from build123d import *

# Parameters (mm, degrees)
EXTRUDE_1_DEPTH = 10
SKETCH_4_W      = 318.818129974
SKETCH_4_H      = 318.818129974
EXTRUDE_3_DEPTH = 20
SKETCH_6_R      = 42
EXTRUDE_4_DEPTH = 85
FILLET_1_R      = 10


with BuildPart() as part:
    # 草图2 → 凸台-拉伸1 (new body)
    with BuildSketch(Plane.XY):
        with BuildLine():
            Line((171.296424673, 156.614258314), (-147.521705301, 156.614258314))
            Line((-147.521705301, 156.614258314), (-147.521705301, -162.20387166))
            Line((-147.521705301, -162.20387166), (171.296424673, -162.20387166))
            Line((171.296424673, -162.20387166), (171.296424673, -121.894806673))
            Line((171.296424673, -121.894806673), (129.887359686, -121.894806673))
            Line((129.887359686, -121.894806673), (129.887359686, -129.352869657))
            Line((129.887359686, -129.352869657), (124.15096929, -129.294806673))
            Line((124.15096929, -129.294806673), (108.887359686, -129.294806673))
            Line((108.887359686, -129.294806673), (108.887359686, -85.749257823))
            ThreePointArc((108.887359686, -85.749257823), (105.533737001, -87.272944854), (101.887359686, -87.794806673))
            Line((101.887359686, -87.794806673), (77.887359686, -87.794806673))
            Line((77.887359686, -87.794806673), (77.887359686, -121.794806673))
            Line((77.887359686, -121.794806673), (-54.112640314, -121.794806673))
            Line((-54.112640314, -121.794806673), (-54.112640314, -87.794806673))
            Line((-54.112640314, -87.794806673), (-78.112640314, -87.794806673))
            ThreePointArc((-78.112640314, -87.794806673), (-87.305028469, -83.987194828), (-91.112640314, -74.794806673))
            Line((-91.112640314, -74.794806673), (-91.112640314, 87.205193327))
            ThreePointArc((-91.112640314, 87.205193327), (-87.305028469, 96.397581483), (-78.112640314, 100.205193327))
            Line((-78.112640314, 100.205193327), (101.887359686, 100.205193327))
            ThreePointArc((101.887359686, 100.205193327), (111.079747841, 96.397581483), (114.887359686, 87.205193327))
            Line((114.887359686, 87.205193327), (114.887359686, -31.294806673))
            Line((114.887359686, -31.294806673), (133.387359686, -31.294806673))
            Line((133.387359686, -31.294806673), (133.387359686, -37.294806673))
            Line((133.387359686, -37.294806673), (133.387359686, -73.794806673))
            Line((133.387359686, -73.794806673), (129.887359686, -73.794806673))
            Line((129.887359686, -73.794806673), (129.887359686, -79.694806673))
            Line((129.887359686, -79.694806673), (171.296424673, -79.694806673))
            Line((171.296424673, -79.694806673), (171.296424673, 156.614258314))
        make_face()
    extrude(amount=EXTRUDE_1_DEPTH)

    # 草图4 → 凸台-拉伸3 (add)
    with BuildSketch(Plane.XY.offset(10)):
        with Locations((11.887359686, -2.794806673)):
            Rectangle(SKETCH_4_W, SKETCH_4_H)
    extrude(amount=EXTRUDE_3_DEPTH)

    # 草图6 → 凸台-拉伸4 (add)
    with BuildSketch(Plane(origin=(0, 0, 10), x_dir=(-1, 0, 0), z_dir=(0, 0, -1))):
        with Locations(Location((-11.887359686, -2.794806673, 0), (0, 0, 180))):
            Circle(SKETCH_6_R)
    extrude(amount=EXTRUDE_4_DEPTH)

    # 圆角1
    fillet_1_edges = [part.edges().sort_by_distance(p)[0] for p in [
        (171.296424673, -162.20387166, 15),
        (-147.521705301, -162.20387166, 15),
        (-147.521705301, 156.614258314, 15),
        (171.296424673, 156.614258314, 15),
    ]]
    fillet(fillet_1_edges, radius=FILLET_1_R)


solid = part.part
Can you work these out from the model? Positions are in its coordinate system, mm. A direction names the side the tool comes from. Coordinates: 2 decimals unless noted, no trailing zeros. Order: outer loops, then holes, each group sorted by start corner. A loop starts at its lowest first (then second) coordinate and runs counter-clockwise, first axis right, second up. Notation, with made-up numbers: (-8.75, 2.5) - (8.25, 2.5) arc R28 cw to (8.25, 31.5) - close; hole circle Ø5 at (-37.5, 75.5). An arc over 180 degrees is marked (long way). Answer as a JSON object with one key per item and string values. Group by question number.
Q1. Imagine slicing it at B-B (x = -66). Please give me the cut outline in (y, z).
Q2. On a 3-axis mill with a long thin cutter (end or side, diameter ignored), from which of +Z, -Z, +X, -X, +Y, -Y can I reach the whole of each face in a straight line? I mean faces 1 (the face through (133.387, -52, 5)), 2 (the face through (168.29, 153.76, 14.79)), 3 (the face through (150, -79.695, 5)). Say none if no direction works.
Q3. Imagine slicing it at A-A (y = 65). Please give me the cut outline in (x, z), and give its area (3 significant figures).
Q4. We'd pull the mould along X, two halves only. Please class faces 4 (the face through (-144.67, 153.61, 14.79)), 5 (the face through (90, -87.795, 5)), 6 (the face through (171.296, -5, 15)), 7 (the face through (151, -121.895, 5)): +X half, -X half, draft (parallel to the pull), parting line (faces both ways), or undercut.
Q5. I need wall thicknesses on line 1 (Y direction, x = 31, z = 6); line 2 (Y direction, x = -74.5, z = 1); line 3 (Z direction, x = 102, y = 64.5). Which ranges of each line are inside material? Lowest first, please. Write a range as from..to.
Q6. Imagine slicing it at C-C (z = -63). Please give me the cut outline in (x, y), and give its area (3 significant figures).
Q7. Will these pins go through, and if not, where does the flat tip stop? P1, Ø12, axis at y = 19, z = -6.5, coming from the -X side; P2, Ø8, axis at x = -66.5, y = 85.5, coming from the -Z side.
Q8. Imagine slicing it at D-D (y = 9). Please give me the cut outline in (x, z).
Determined:
{
 "1": {"outline": "(-162.2, 0) - (-87.79, 0) - (-87.79, 10) - (100.21, 10) - (100.21, 0) - (156.61, 0) - (156.61, 30) - (-162.2, 30) - close"},
 "2": {"face 1": "-Z", "face 2": "+Z, -Z, +X, +Y", "face 3": "-Z, +X"},
 "3": {"outline": "(-147.52, 0) - (-91.11, 0) - (-91.11, 10) - (114.89, 10) - (114.89, 0) - (171.3, 0) - (171.3, 30) - (-147.52, 30) - close", "area": "7,500 mm2"},
 "4": {"face 4": "-X half", "face 5": "undercut", "face 6": "+X half", "face 7": "draft"},
 "5": {"line 1": "y = -162.2..-121.79, -40.19..34.6, 100.21..156.61", "line 2": "y = -162.2..-87.79, 100.21..156.61", "line 3": "z = 10..30"},
 "6": {"outline": "circle Ø84 at (11.89, -2.79)", "area": "5,540 mm2"},
 "7": {"P1": "stops at x = -27.03", "P2": "stops at z = 10"},
 "8": {"outline": "(-147.52, 0) - (-91.11, 0) - (-91.11, 10) - (-28.42, 10) - (-28.42, -75) - (52.2, -75) - (52.2, 10) - (114.89, 10) - (114.89, 0) - (171.3, 0) - (171.3, 30) - (-147.52, 30) - close"}
}
